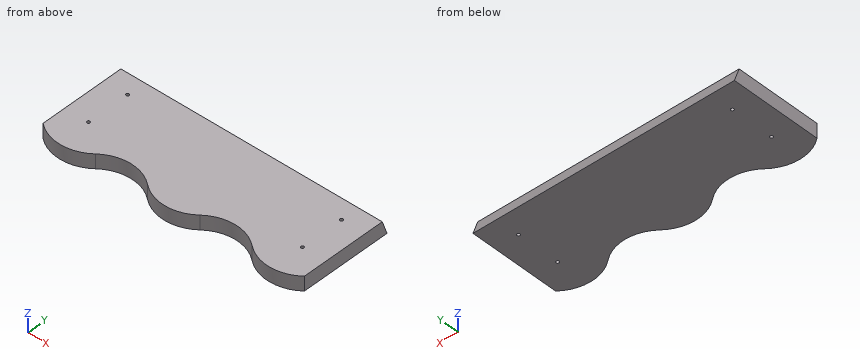
from build123d import *

# Parameters (mm, degrees)
F0_R     = 2.032
F1_DEPTH = 19.05
F3_DEPTH = 349.25


with BuildPart() as f1:
    # F0 (on Top) → F1 (new body)
    with BuildSketch(Plane.XY):
        with BuildLine():
            Line((174.625, -53.986043), (174.625, 66.675))
            Line((174.625, 66.675), (-174.625, 66.675))
            Line((-174.625, 66.675), (-174.625, -53.986043))
            ThreePointArc((-174.625, -53.986043), (-139.7, -66.67541), (-104.775, -53.986043))
            ThreePointArc((-104.775, -53.986043), (-69.85, -41.296677), (-34.925, -53.986043))
            ThreePointArc((-34.925, -53.986043), (0, -66.675), (34.925, -53.986043))
            ThreePointArc((34.925, -53.986043), (69.85, -41.296677), (104.775, -53.986043))
            ThreePointArc((104.775, -53.986043), (139.7, -66.67541), (174.625, -53.986043))
        make_face()
        with Locations((-142.875, -22.225)):
            Circle(F0_R, mode=Mode.SUBTRACT)
        with Locations((142.875, -22.225)):
            Circle(F0_R, mode=Mode.SUBTRACT)
        with Locations((-142.875, 34.925)):
            Circle(F0_R, mode=Mode.SUBTRACT)
        with Locations((142.875, 34.925)):
            Circle(F0_R, mode=Mode.SUBTRACT)
    extrude(amount=F1_DEPTH)

    # F2 (on face) → F3 (cut)
    with BuildSketch(Plane(origin=(-174.625, 0, 0), x_dir=(0, -1, 0), z_dir=(-1, 0, 0))):
        Polygon((-59.741367, 19.05), (-66.675, 19.05), (-66.675, 0), align=None)
    extrude(amount=-F3_DEPTH, mode=Mode.SUBTRACT)


solid = f1.part
Source: CAD feature listing. Evaluate the final solid. Frame: model axes, mm. Give positions to 0.01 mm unless a question says otherwise; leave off trailing zeros. Write each loop counter-clockwise with the first axis right and the second up, starting at its lowest first coordinate (ties: lowest second). Pieces come first, ordered by that corner, then holes. Notation, with made-up numbers: M -29.75,17.25 L 5.25,17.25 A32 ccw 5.25,51.25 Z; hole C 21,30 d4. An arc over 180 degrees is marked long. Return JSON: item names as keys, results as strings. Group by question number.
1) Cut plane A-A, the plane y = -45. Output: boundary loops of the cut face in (x, z) (3 decimals).
2) Cut plane B-B, the plane z = 3.5. Output: boundary loops of the cut face in (x, y) (3 decimals).
3) Material intervals for line 1 along X through (y, z) = (35, 8.25) (3 decimals); line 2 along X through (y, z) = (-61, 4.25); line 3 along Y through (x, z) = (-156, 14.25), sorted ascending. Write a range as [from, to].
4) Cut plane C-C, the plane x = -114.5. Output: boundary loops of the cut face in (y, z) (3 decimals), plus the area to 3 significant figures.
5) Cut plane D-D, the plane x = 16. Output: boundary loops of the cut face in (y, z) (3 decimals), plus the area to 3 significant figures.
6) Pin query (flat end, axial travel): P1, Ø5, axis at x = -11, z = 9.5, coming from the -Y side; P2, Ø2, axis at x = 18.5, z = 12.5, coming from the -Y side; P3, Ø5, axis at x = 4, z = 10, coming from the -Y side. Return the tip coordinate at first contact, or that it passes through.
Recorded:
{
 "1": {"outline": "M -174.625,0 L -89.58,0 L -89.58,19.05 L -174.625,19.05 Z; M -50.12,0 L 50.12,0 L 50.12,19.05 L -50.12,19.05 Z; M 89.58,0 L 174.625,0 L 174.625,19.05 L 89.58,19.05 Z"},
 "2": {"outline": "M -174.625,-53.986 A54.407 ccw -104.775,-53.986 A54.407 cw -34.925,-53.986 A54.408 ccw 34.925,-53.986 A54.407 cw 104.775,-53.986 A54.407 ccw 174.625,-53.986 L 174.625,65.401 L -174.625,65.401 Z; hole C -142.875,-22.225 d4.064; hole C -142.875,34.925 d4.064; hole C 142.875,-22.225 d4.064; hole C 142.875,34.925 d4.064"},
 "3": {"line 1": "x = [-174.625, -144.906], [-140.844, 140.844], [144.906, 174.625]", "line 2": "x = [-163.89, -115.51], [-24.19, 24.19], [115.51, 163.89]", "line 3": "y = [-64.18, 61.49]"},
 "4": {"outline": "M -60.487,0 L 66.675,0 L 59.741,19.05 L -60.487,19.05 Z", "area": "2,360 mm²"},
 "5": {"outline": "M -64.269,0 L 66.675,0 L 59.741,19.05 L -64.269,19.05 Z", "area": "2,430 mm²"},
 "6": {"P1": "stops at y = -66.01", "P2": "stops at y = -63.78", "P3": "stops at y = -66.65"}
}
